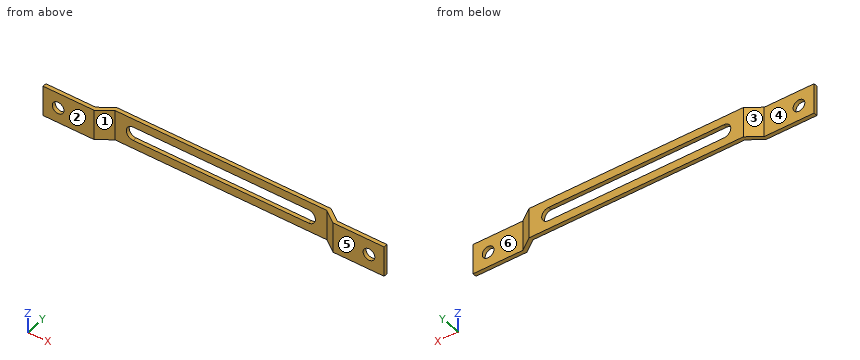
```python
from build123d import *

# Parameters (mm, degrees)
EXTRUDE_1_DEPTH     = 15.5
SKETCH_2_R          = 3
CUT_EXTRUDE_1_DEPTH = 10


with BuildPart() as part:
    # Эскиз1 → Вытянуть-Тонкостенный1 (new body)
    with BuildSketch(Plane.XY):
        Polygon((87.5, 0), (61.92820323, 0), (55, 5), (-55, 5), (-61.92820323, 0), (-87.5, 0), (-87.5, -2), (-61.281883024, -2), (-54.353679794, 3), (54.353679794, 3), (61.281883024, -2), (87.5, -2), align=None)
    extrude(amount=EXTRUDE_1_DEPTH)

    # Эскиз2 → Вырез-Вытянуть1 (cut)
    with BuildSketch(Plane(origin=(0, 5, 0), x_dir=(1, 0, 0), z_dir=(0, 1, 0))):
        with Locations((-79.75, -7.75)):
            Circle(SKETCH_2_R)
        with Locations((79.75, -7.75)):
            Circle(SKETCH_2_R)
        with BuildLine():
            Line((-45, -4.25), (45, -4.25))
            ThreePointArc((45, -4.25), (48.5, -7.75), (45, -11.25))
            Line((45, -11.25), (-45, -11.25))
            ThreePointArc((-45, -11.25), (-48.5, -7.75), (-45, -4.25))
        make_face()
    extrude(amount=-CUT_EXTRUDE_1_DEPTH, mode=Mode.SUBTRACT)


solid = part.part
```
Can you work these out from the model? Positions are in its coordinate system, mm. Face numbers are marked on the shaded views. A direction names the side the tool comes from. Coordinates: 2 decimals unless noted, no trailing zeros. Loops run counter-clockwise (first coordinate to the right, second up) from the corner with the lowest first, then second, coordinate; pieces in that order, holes last.
Item 1: If we mould it in two halves opening along X, with no side actions, what happens to the marked faces 1, 2 and 3? For each: released by +X, released by -X, zero draft, split by the parting line, or undercut.
Answers below:
face 1: undercut
face 2: zero draft
face 3: released by -X
Item 2: Please list where these lines run through material, in increasing order: L1, parallel to X at y = -1.55, z = 7.75; L2, parallel to Z at x = -79.75, y = -0.8; L3, parallel to X at y = -0.5, z = 8.5.
Answers below:
L1: x = -87.5 to -82.75, -76.75 to -60.66, 60.66 to 76.75, 82.75 to 87.5
L2: z = 0 to 4.75, 10.75 to 15.5
L3: x = -87.5 to -82.65, -76.85 to -59.2, 59.2 to 76.85, 82.65 to 87.5
Item 3: Which directions (+Z, -Z, +X, -X, +Y, -Y) give clear straight access to the entire face, cutting with the end or side of a thin tool? Please do the marked faces 4, 5 and 6.
Answers below:
face 4: +Z, -Z, -X, +Y
face 5: +Z, -Z, +X, -X, -Y
face 6: +Z, -Z, +X, +Y
Item 4: Suppose I cut it at B-B (z = 7.75). Please give me the cut outline in (x, y), then the cut area to 3 significant figures.
Answers below:
outline: (-87.5, -2) - (-82.75, -2) - (-82.75, 0) - (-87.5, 0) - close; (-76.75, -2) - (-61.28, -2) - (-54.35, 3) - (-48.5, 3) - (-48.5, 5) - (-55, 5) - (-61.93, 0) - (-76.75, 0) - close; (48.5, 3) - (54.35, 3) - (61.28, -2) - (76.75, -2) - (76.75, 0) - (61.93, 0) - (55, 5) - (48.5, 5) - close; (82.75, -2) - (87.5, -2) - (87.5, 0) - (82.75, 0) - close
area: 138 mm2
Item 5: I'm going to push flat-ended pins straight in: pin 1 (5 mm diameter, centred on x = -79.75, z = 7.75, fed in from -Y); pin 2 (4.5 mm diameter, centred on x = -77.5, z = 6.5, fed in from +Y); pin 3 (2 mm diameter, centred on x = 8.5, z = 10.5, fed in from -Y); pin 4 (2 mm diameter, centred on x = -13, y = 4, fed in from -Z). Where does each tip first touch, or does it pass through?
Answers below:
pin 1: passes through
pin 2: stops at y = 0
pin 3: stops at y = 3
pin 4: stops at z = 0
Item 6: Suppose I cut it at A-A (x = 79.75). Please give me the cut outline in (y, z).
Answers below:
outline: (-2, 0) - (0, 0) - (0, 4.75) - (-2, 4.75) - close; (-2, 10.75) - (0, 10.75) - (0, 15.5) - (-2, 15.5) - close
Item 7: Suppose I cut it at C-C (x = -21). Please give me the cut outline in (y, z).
Answers below:
outline: (3, 0) - (5, 0) - (5, 4.25) - (3, 4.25) - close; (3, 11.25) - (5, 11.25) - (5, 15.5) - (3, 15.5) - close
